from build123d import *

# Parameters (mm, degrees)
SKETCH1_R                    = 150
BOSS_EXTRUDE1_DEPTH          = 75
CHAMFER1_SIZE                = 10
BOSS_EXTRUDE2_DEPTH          = 10
CHAMFER2_SIZE                = 7
BOSS_EXTRUDE3_DEPTH          = 9
BOSS_EXTRUDE4_DEPTH          = 3.5
CIRPATTERN1_COUNT            = 4
CIRPATTERN1_COPY_1_DEPTH     = 9
CIRPATTERN1_COPY_2_DEPTH     = 9
CIRPATTERN1_COPY_3_DEPTH     = 9
CIRPATTERN1_COPY_4_DEPTH     = 3.5
CIRPATTERN1_COPY_5_DEPTH     = 3.5
CIRPATTERN1_COPY_6_DEPTH     = 3.5
CHAMFER2_OF_CIRPATTERN1_SIZE = 7
SKETCH5_R                    = 110
BOSS_EXTRUDE5_DEPTH          = 9
BOSS_EXTRUDE5_TAPER          = 45
CUT_EXTRUDE1_START           = -60
CUT_EXTRUDE1_DEPTH           = 60
SKETCH7_R                    = 15
BOSS_EXTRUDE6_DEPTH          = 20
SKETCH8_R                    = 27.5
CUT_EXTRUDE2_DEPTH           = 60


with BuildPart() as part:
    # Sketch1 → Boss-Extrude1 (new body)
    with BuildSketch(Plane(origin=(0, 0, 0), x_dir=(1, 0, 0), z_dir=(0, 1, 0))):
        with Locations(Location((0, 0, 0), (0, 0, 270))):
            Circle(SKETCH1_R)
    extrude(amount=BOSS_EXTRUDE1_DEPTH)

    # Chamfer1
    chamfer1_edges = [part.edges().sort_by_distance(p)[0] for p in [
        (0, 75, -150),
    ]]
    chamfer(chamfer1_edges, length=CHAMFER1_SIZE)

    # Sketch2 → Boss-Extrude2 (add)
    with BuildSketch(Plane.XZ):
        with BuildLine():
            Line((145.236875483, 37.5), (195.236875483, 37.5))
            Line((195.236875483, 37.5), (195.236875483, -37.5))
            Line((195.236875483, -37.5), (145.236875483, -37.5))
            ThreePointArc((145.236875483, -37.5), (150, 0), (145.236875483, 37.5))
        make_face()
    boss_extrude2 = extrude(amount=-BOSS_EXTRUDE2_DEPTH)

    # Chamfer2
    chamfer2_edges = [part.edges().sort_by_distance(p)[0] for p in [
        (195.236875483, 5, 37.5),
        (195.236875483, 5, -37.5),
    ]]
    chamfer(chamfer2_edges, length=CHAMFER2_SIZE)

    # Sketch3 → Boss-Extrude3 (add)
    with BuildSketch(Plane(origin=(0, 0, -37.5), x_dir=(-1, 0, 0), z_dir=(0, 0, -1))):
        Polygon((-145.236875483, 10), (-145.236875483, 65), (-170.556875483, 65), (-188.236875483, 10), align=None)
    boss_extrude3 = extrude(amount=-BOSS_EXTRUDE3_DEPTH)

    # Sketch4 → Boss-Extrude4 (add)
    with BuildSketch(Plane(origin=(0, 10, 0), x_dir=(1, 0, 0), z_dir=(0, 1, 0))):
        Polygon((188.236875483, 21), (183.04072306, 18), (183.04072306, 12), (188.236875483, 9), (193.433027905, 12), (193.433027905, 18), align=None)
    boss_extrude4 = extrude(amount=BOSS_EXTRUDE4_DEPTH)

    # Mirror1: Boss-Extrude3, Boss-Extrude4 across plane
    add(boss_extrude3.mirror(Plane.XY))
    add(boss_extrude4.mirror(Plane.XY))

    # CirPattern1: Boss-Extrude2, Boss-Extrude3, Boss-Extrude4 ×4 about axis
    cirpattern1_axis = Axis((0, 0, 0), (0, 1, 0))
    add([boss_extrude2.rotate(cirpattern1_axis, i * 360 / CIRPATTERN1_COUNT) for i in range(1, CIRPATTERN1_COUNT)])
    add([boss_extrude3.rotate(cirpattern1_axis, i * 360 / CIRPATTERN1_COUNT) for i in range(1, CIRPATTERN1_COUNT)])
    add([boss_extrude4.rotate(cirpattern1_axis, i * 360 / CIRPATTERN1_COUNT) for i in range(1, CIRPATTERN1_COUNT)])

    # CirPattern1 copy 1 sketch → CirPattern1 copy 1 (add)
    with BuildSketch(Plane(origin=(37.5, 0, 0), x_dir=(0, 0, 1), z_dir=(1, 0, 0))):
        Polygon((-145.236875483, -10), (-145.236875483, -65), (-170.556875483, -65), (-188.236875483, -10), align=None)
    extrude(amount=-CIRPATTERN1_COPY_1_DEPTH)

    # CirPattern1 copy 2 sketch → CirPattern1 copy 2 (add)
    with BuildSketch(Plane(origin=(0, 0, -37.5), x_dir=(1, 0, 0), z_dir=(0, 0, -1))):
        Polygon((-145.236875483, -10), (-145.236875483, -65), (-170.556875483, -65), (-188.236875483, -10), align=None)
    extrude(amount=-CIRPATTERN1_COPY_2_DEPTH)

    # CirPattern1 copy 3 sketch → CirPattern1 copy 3 (add)
    with BuildSketch(Plane(origin=(-37.5, 0, 0), x_dir=(0, 0, -1), z_dir=(-1, 0, 0))):
        Polygon((-145.236875483, -10), (-145.236875483, -65), (-170.556875483, -65), (-188.236875483, -10), align=None)
    extrude(amount=-CIRPATTERN1_COPY_3_DEPTH)

    # CirPattern1 copy 4 sketch → CirPattern1 copy 4 (add)
    with BuildSketch(Plane(origin=(0, 10, 0), x_dir=(0, 0, -1), z_dir=(0, 1, 0))):
        Polygon((188.236875483, -21), (183.04072306, -18), (183.04072306, -12), (188.236875483, -9), (193.433027905, -12), (193.433027905, -18), align=None)
    extrude(amount=CIRPATTERN1_COPY_4_DEPTH)

    # CirPattern1 copy 5 sketch → CirPattern1 copy 5 (add)
    with BuildSketch(Plane(origin=(0, 10, 0), x_dir=(-1, 0, 0), z_dir=(0, 1, 0))):
        Polygon((188.236875483, -21), (183.04072306, -18), (183.04072306, -12), (188.236875483, -9), (193.433027905, -12), (193.433027905, -18), align=None)
    extrude(amount=CIRPATTERN1_COPY_5_DEPTH)

    # CirPattern1 copy 6 sketch → CirPattern1 copy 6 (add)
    with BuildSketch(Plane.ZX.offset(10)):
        Polygon((188.236875483, -21), (183.04072306, -18), (183.04072306, -12), (188.236875483, -9), (193.433027905, -12), (193.433027905, -18), align=None)
    extrude(amount=CIRPATTERN1_COPY_6_DEPTH)

    # Chamfer2 of CirPattern1
    chamfer2_of_cirpattern1_edges = [part.edges().sort_by_distance(p)[0] for p in [
        (37.5, 5, -195.236875483),
        (-37.5, 5, -195.236875483),
        (-195.236875483, 5, -37.5),
        (-195.236875483, 5, 37.5),
        (-37.5, 5, 195.236875483),
        (37.5, 5, 195.236875483),
    ]]
    chamfer(chamfer2_of_cirpattern1_edges, length=CHAMFER2_OF_CIRPATTERN1_SIZE)

    # Sketch5 → Boss-Extrude5 (add)
    with BuildSketch(Plane(origin=(0, 75, 0), x_dir=(1, 0, 0), z_dir=(0, 1, 0))):
        Circle(SKETCH5_R)
    extrude(amount=BOSS_EXTRUDE5_DEPTH, taper=BOSS_EXTRUDE5_TAPER)

    # Sketch6 → Cut-Extrude1 (cut)
    with BuildSketch(Plane(origin=(0, 75, 0), x_dir=(1, 0, 0), z_dir=(0, 1, 0)).offset(CUT_EXTRUDE1_START)):
        with BuildLine():
            Line((-112.583302492, -65), (-129.903810568, -75))
            ThreePointArc((-129.903810568, -75), (-106.066017178, -106.066017178), (-75, -129.903810568))
            Line((-75, -129.903810568), (-65, -112.583302492))
            ThreePointArc((-65, -112.583302492), (-91.923881554, -91.923881554), (-112.583302492, -65))
        make_face()
    extrude(amount=CUT_EXTRUDE1_DEPTH, mode=Mode.SUBTRACT)

    # Sketch7 → Boss-Extrude6 (add)
    with BuildSketch(Plane(origin=(0, 84, 0), x_dir=(1, 0, 0), z_dir=(0, 1, 0))):
        with Locations(Location((0, 0, 0), (0, 0, 270))):
            Circle(SKETCH7_R)
    extrude(amount=BOSS_EXTRUDE6_DEPTH)

    # Sketch8 → Cut-Extrude2 (cut)
    with BuildSketch(Plane.XZ):
        with Locations(Location((0, 0, 0), (0, 0, 270))):
            Circle(SKETCH8_R)
    extrude(amount=-CUT_EXTRUDE2_DEPTH, mode=Mode.SUBTRACT)


solid = part.part
Work out the finished part from the listing and answer in its coordinate system (mm). A direction names the side the tool comes from. Round coordinates to 2 decimals unless told otherwise and drop trailing zeros. Write each loop counter-clockwise with the first axis right and the second up, starting at its lowest first coordinate (ties: lowest second). Pieces come first, ordered by that corner, then holes. Notation, with made-up numbers: (78.5, -20.75) - (85.5, -20.75) arc R33 cw to (85.5, 7.25) - close; hole circle Ø2 at (-3, 14). An arc over 180 degrees is marked (long way). Answer in a Markdown table with one row per item. Add a question column.
1. A cutting plane is placed at B-B, the plane y = 93.5. Determine the outline of the cut face in (x, z), and give its area (3 significant figures).
2. Find the intervals of material crossed by line 1 along X through (y, z) = (50, -155); line 2 along X through (y, z) = (23, 0); line 3 along Y through (x, z) = (-50, -20), in increasing order. Write a range as from..to.
3. For faces 4 (the flat face through (-37.5, 32, 162)), 5 (the flat face through (37.5, 32, 162)), 6 (the flat face through (-188, 13.5, 15)), 7 (the cylindrical face through (0.66, 93.86, -14.985)), determine the directions among +Z, -Z, +X, -X, +Y, -Y from which every point of the face is accessible in a straight line to the end or side of a thin tool.
4. Given pin 1 (7 mm diameter, centred on x = -31, z = 151.5, fed in from +Y); pin 2 (1 mm diameter, centred on y = 11.5, z = 14, fed in from -X); pin 3 (2 mm diameter, centred on x = 138.5, y = 51, fed in from -Z), each flat-ended and moving along its own axis, determine where each tip first touches the part or whether it passes through.
5. A cutting plane is placed at A-A, the plane x = 0. Determine the outline of the cut face in (y, z), and give its area (3 significant figures).
6. The mould has two halves that part along Z. Classify faces 1 (the flat face through (-121.12, 44.58, 69.93)), 2 (the cylindrical face through (-91.586, 44.58, 92.26)), 3 (the flat face through (-72, 75, -84)): +Z half, -Z half, draft (parallel to the pull), parting line (faces both ways), or undercut.
Worked out:
| question | item | result |
|---|---|---|
| 1 | outline | circle Ø30 at (0, 0) |
| 1 | area | 707 mm^2 |
| 2 | line 1 | -37.5..-28.5, 28.5..37.5 |
| 2 | line 2 | -150..-27.5, 27.5..150 |
| 2 | line 3 | 0..84 |
| 3 | face 4 | +Z, -X, +Y, -Y |
| 3 | face 5 | +Z, +X, +Y, -Y |
| 3 | face 6 | -X, +Y |
| 3 | face 7 | +Y |
| 4 | pin 1 | y = 65 |
| 4 | pin 2 | x = -193.43 |
| 4 | pin 3 | z = -59.95 |
| 5 | outline | (0, -195.24) - (10, -195.24) - (10, -150) - (65, -150) - (75, -140) - (75, -110) - (84, -101) - (84, -15) - (104, -15) - (104, 15) - (84, 15) - (84, 101) - (75, 110) - (75, 140) - (65, 150) - (10, 150) - (10, 195.24) - (0, 195.24) - (0, 27.5) - (60, 27.5) - (60, -27.5) - (0, -27.5) - close |
| 5 | area | 22,500 mm^2 |
| 6 | face 1 | +Z half |
| 6 | face 2 | undercut |
| 6 | face 3 | draft |
